Autodesk Inventor part; units mm, degrees
ref_plane "YZ Plane" through (0, 0, 0) normal (1, 0, 0) x (0, 1, 0)
ref_plane "XZ Plane" through (0, 0, 0) normal (0, 1, 0) x (-1, 0, 0)
ref_plane "XY Plane" through (0, 0, 0) normal (0, 0, 1) x (1, 0, 0)
sketch "Skizze3" plane through (0, 0, 0) normal (0, 0, 1) x (1, 0, 0)
  line L0 (0, 0) -> (-40, 0)
  line L1 (-40, 0) -> (-40, 35)
  line L2 (-40, 35) -> (0, 35)
  line L3 (0, 35) -> (0, 0)
  point P0 (-3.7, 3.7)
  dimension "d4" = 35
  dimension "d5" = 40
  dimension "d6" = 3.7
  dimension "d7" = 3.7
sketch "Skizze4" plane through (0, 0, 0) normal (0, 1, 0) x (-1, 0, 0)
  line L0 (0, 0) -> (40, 0)
  line L1 (20, 0) -> (20, 25)
  line L2 (20, 18) -> (20, 12) construction
  line L3 (24, 18) -> (24, 12)
  line L4 (16, 12) -> (16, 18)
  arc A0 (24, 18) -> (16, 18) centre (20, 18) ccw
  arc A1 (16, 12) -> (24, 12) centre (20, 12) ccw
  circle A2 centre (20, 15) radius 10
  line L5 (30, 15) -> (30, 0)
  line L6 (10, 15) -> (10, 0)
  dimension "d9" = 10
  dimension "d10" = 8
  dimension "d11" = 6
  dimension "d12" = 10
  dimension "d13" = 10
  dimension "d46" = 12
extrude "Extrusion3" add sketch "Skizze4" along normal blind 35 contours L6 A2 L1 L0 | L1 A2 L5 L0 | A2 L1 A0 L4 A1 | L1 A1 L3 A0 A2
extrude "Extrusion4" add sketch "Skizze3" against normal blind 3
hole "Bohrung1" at (-3.7, 3.7, 0) direction (0, 0, -1) diameter 2.459 depth 8.8 countersink diameter 7 countersink angle 90
sketch "Skizze5" plane through (0, 0, 0) normal (1, 0, 0) x (0, 0, -1)
  line L0 (-25, 0) -> (-25, 35)
  line L1 (-25, 8.1) -> (0, 8.1)
  line L2 (0, 8.1) -> (0, 26.9)
  line L3 (0, 26.9) -> (-25, 26.9)
  line L4 (-25, 26.9) -> (-25, 8.1)
  line L5 (0, 0) -> (0, 35)
  point P0 (-25, 17.5)
  point P1 (-25, 26.9)
  point P2 (0, 17.5)
  point P3 (0, 17.5)
  dimension "d25" = 18.8
extrude "Extrusion5" cut sketch "Skizze5" against normal through all
pattern_linear "Rechteckige Anordnung1" count 2 spacing 32.6 along (-1, 0, 0) count 2 spacing 27.6 along (0, 1, 0) of "Bohrung1"
sketch "Skizze6" plane through (-20, 26.9, 15) normal (0, -1, 0) x (1, 0, 0)
  line L0 (-10, -15) -> (-10, 0)
  line L1 (10, 0) -> (10, -15)
  line L2 (10, -15) -> (-10, -15)
  arc A0 (-4, -3) -> (4, -3) centre (0, -3) ccw
  arc A1 (10, 0) -> (-10, 0) centre (0, 0) ccw
  line L3 (10, 0) -> (10, -15)
  line L4 (-10, -15) -> (-10, 0)
  circle A2 centre (0, -3) radius 11.5
  line L5 (-6.6647, -12.3719) -> (-10, -10)
  line L6 (10, 0) -> (10, -15)
  line L7 (10, -10) -> (6.6647, -12.3719)
  point P0 (20, -15)
  point P1 (-10, -10)
  dimension "d47" = 23
  dimension "d48" = 5
  dimension "d49" = 5
extrude "Extrusion6" add sketch "Skizze6" along normal up to surface (18.8 mm away) contours L0 L5 A2 L7 L1 L2
fillet "Rundung4" radius 2 2 edges at (-10, 17.5, 0) (-30, 17.5, 0)
fillet "Rundung5" radius 0.2 2 edges at (-30, 17.5, 5) (-10, 17.5, 5)
equation "\"d13\" = d12"
equation "\"d14\" = d4"
equation "\"d31\" = d5 - 2 * d6"
equation "\"d34\" = d4 - 2 * d7"
properties part number "BT101_trajan20_21" material "Kunststoff, undurchsichtig Schwarz"
Input: part model. Units: mm. Frame: model coordinates. A direction names the side the tool comes from. Coordinates: 2 decimals unless noted, no trailing zeros. Loops run counter-clockwise (first coordinate to the right, second up) from the corner with the lowest first, then second, coordinate; pieces in that order, holes last. Notation, with made-up numbers: (56.25, 26.25) - (88.25, 26.25) arc R22 ccw to (88.25, 35.25) - close; hole circle Ø6 at (40.25, 82). An arc over 180 degrees is marked (long way). Answer in a Markdown table with one row per item. Add a question column.
Item 1: Mould query, pull axis Y, two halves, no side actions, for faces 1 (the flat face through (-20, 35, 5)), 2 (the flat face through (-20, 0, 5)), 3 (the cylindrical face through (-35.21, 30.73, -2.64)), 4 (the cylindrical face through (-20, 31, 8)). Classes: released by +Y, released by -Y, zero draft, split by the parting line, or undercut.
Item 2: Section query B-B on y = 3.7. Return the cut outline in (x, z).
Item 3: Section query A-A on x = -20. Return the cut outline in (y, z), then the cut area to 3 significant figures.
Item 4: Section query D-D on x = -36.3. Return the cut outline in (y, z).
Item 5: Section query C-C on z = 9. Return the cut outline in (x, y), then the cut area to 3 significant figures.
Item 6: Access query for faces 5 (the flat face through (-20, 26.9, 7)), 6 (the flat face through (-16, 31, 15)), 7 (the flat face through (-10, 17, 4)). Directions: +Z, -Z, +X, -X, +Y, -Y. A direction counts if a zero-diameter tool reaches every point of the face in a straight line with its end or side. Return the directions, or none.
Item 7: Contact query for flat-ended pins moving along their axis: P1, Ø1.8, axis at y = 4.5, z = 15, coming from the +X side; P2, Ø5, axis at y = 6, z = 16.5, coming from the -X side; P3, Ø6.5, axis at x = -38, y = 20.5, coming from the +Z side. Output: stop coordinate, or through.
Item 8: Line query: line 1 along X through (y, z) = (31.3, -2.8); line 2 along Y through (x, z) = (-3.7, -2.8); line 3 along Y through (x, z) = (-24, 4.25). Output: solid intervals per line, ascending. Write a range as [from, to].
Recorded:
| question | item | result |
|---|---|---|
| 1 | face 1 | released by +Y |
| 1 | face 2 | released by -Y |
| 1 | face 3 | undercut |
| 1 | face 4 | zero draft |
| 2 | outline | (-40, -3) - (-37.53, -3) - (-37.53, -2.27) - (-39.8, 0) - (-40, 0) - close; (-35.07, -3) - (-4.93, -3) - (-4.93, -2.27) - (-7.2, 0) - (-8, 0) arc R2 cw to (-10, 2) - (-10, 15) arc R10 ccw to (-30, 15) - (-30, 2) arc R2 cw to (-32, 0) - (-32.8, 0) - (-35.07, -2.27) - close; (-2.47, -3) - (0, -3) - (0, 0) - (-0.2, 0) - (-2.47, -2.27) - close; hole (-24, 12) arc R4 ccw to (-16, 12) - (-16, 18) arc R4 ccw to (-24, 18) - close |
| 3 | outline | (0, -3) - (35, -3) - (35, 8) - (26.9, 8) - (26.9, 0.5) - (8.1, 0.5) - (8.1, 8) - (0, 8) - close; (0, 22) - (8.1, 22) - (8.1, 25) - (0, 25) - close; (26.9, 22) - (35, 22) - (35, 25) - (26.9, 25) - close |
| 3 | area | 293 mm^2 |
| 4 | outline | (0, -3) - (2.47, -3) - (2.47, -2.27) - (0.2, 0) - (0, 0) - close; (4.93, -3) - (30.07, -3) - (30.07, -2.27) - (27.8, 0) - (7.2, 0) - (4.93, -2.27) - close; (32.53, -3) - (35, -3) - (35, 0) - (34.8, 0) - (32.53, -2.27) - close |
| 5 | outline | (-30, 0) - (-22.65, 0) - (-22.65, 8.1) - (-30, 8.1) - close; (-30, 26.9) - (-22.65, 26.9) - (-22.65, 35) - (-30, 35) - close; (-17.35, 0) - (-10, 0) - (-10, 8.1) - (-17.35, 8.1) - close; (-17.35, 26.9) - (-10, 26.9) - (-10, 35) - (-17.35, 35) - close |
| 5 | area | 238 mm^2 |
| 6 | face 5 | +Z |
| 6 | face 6 | +Y, -Y |
| 6 | face 7 | +Z, +X, +Y, -Y |
| 7 | P1 | x = -10 |
| 7 | P2 | x = -30 |
| 7 | P3 | z = 0 |
| 8 | line 1 | [-40, -37.53], [-35.07, -4.93], [-2.47, 0] |
| 8 | line 2 | [0, 2.47], [4.93, 30.07], [32.53, 35] |
| 8 | line 3 | [0, 8.1], [26.9, 35] |
